Geometry check sheet. Reference: the model listing, model coordinates, mm. A direction names the side the tool comes from. Coordinates: 2 decimals unless noted, no trailing zeros. Write each loop counter-clockwise with the first axis right and the second up, starting at its lowest first coordinate (ties: lowest second). Pieces come first, ordered by that corner, then holes. Notation, with made-up numbers: (61.5, 75.5) -> (118.5, 75.5) arc R12 ccw to (118.5, 86.5) -> close; hole circle Ø3 at (63.5, -11). An arc over 180 degrees is marked (long way). Answer in a Markdown table with one row per item. Add a question column.
1. Cross-section at A-A on y = -35. Record the cut outline in (x, z).
2. Set-up check for faces 5 (the flat face through (0.737, -25, 30)), 6 (the flat face through (-1, -25, 16.398)), 7 (the flat face through (1, 0, 24)): record each of +Z, -Z, +X, -X, +Y, -Y from which the full face is reachable in a straight line by a thin tool's end or side.
3. Cross-section at D-D on x = -4. Record the cut outline in (y, z).
4. Cross-section at B-B on x = -7. Record the cut outline in (y, z).
5. Mould release check, pull along X, two halves, no side actions. Record for faces 1 (the flat face through (-6.263, -25, 5)), 2 (the cylindrical face through (-4.833, -14.549, 40.919)), 3 (the flat face through (-4, -25, 39.398)), 4 (the cylindrical face through (-6.589, -36.464, 40.919)): pulls with the +X half, pulls with the -X half, needs draft (parallel to the pull), parting line crosses it, or undercut.
6. Depth check by flat-ended pin: P1, Ø1.5, axis at y = -25, z = 36.5, coming from the -X side; P2, Ø2, axis at x = 1, y = -13, coming from the -Z side; P3, Ø2, axis at x = -4.5, z = 3, coming from the -Y side; P4, Ø18.5, axis at y = -27.5, z = 2, coming from the +X side. Enter the tip coordinate at first touch or a pass-through.
7. Cross-section at C-C on z = 5.5. Record the cut outline in (x, y).
8. Scan lines: L1, parallel to Z at x = -8.5, y = -35; L2, parallel to Z at x = -7.55, y = -15; L3, parallel to Z at x = -5, y = -9.5. Record each from-to range of solid material in increasing order. Write a range as from..to.
```python
from build123d import *

# Parameters (mm, degrees)
F1_DEPTH = 50
F2_R     = 1.5
F3_DEPTH = 10
F4_R     = 1.5
F5_DEPTH = 25


with BuildPart() as f1:
    # F0 (on Front) → F1 (new body)
    with BuildSketch(Plane.XZ):
        Polygon((-9.26335, 42.398173), (-9.26335, 39.398173), (0.73665, 39.398173), (0.73665, 19.398173), (-9.26335, 19.398173), (-9.26335, -6.901827), (-6.26335, -6.901827), (-6.26335, 16.398173), (3.73665, 16.398173), (3.73665, 42.398173), align=None)
    extrude(amount=F1_DEPTH)

    # F2 (on face) → F3 (cut)
    with BuildSketch(Plane.XY.offset(42.398173)):
        with Locations((-6.26335, -35)):
            Circle(F2_R)
        with Locations((-6.26335, -15)):
            Circle(F2_R)
    extrude(amount=-F3_DEPTH, mode=Mode.SUBTRACT)

    # F4 (on face) → F5 (cut)
    with BuildSketch(Plane.YZ.offset(-6.26335)):
        with Locations((-35, 6.098173)):
            Circle(F4_R)
        with Locations((-15, 6.098173)):
            Circle(F4_R)
    extrude(amount=-F5_DEPTH, mode=Mode.SUBTRACT)


solid = f1.part
```
Results found:
| question | item | result |
|---|---|---|
| 1 | outline | (-9.26, -6.9) -> (-6.26, -6.9) -> (-6.26, 4.6) -> (-9.26, 4.6) -> close; (-9.26, 7.6) -> (-6.26, 7.6) -> (-6.26, 16.4) -> (3.74, 16.4) -> (3.74, 42.4) -> (-4.76, 42.4) -> (-4.76, 39.4) -> (0.74, 39.4) -> (0.74, 19.4) -> (-9.26, 19.4) -> close; (-9.26, 39.4) -> (-7.76, 39.4) -> (-7.76, 42.4) -> (-9.26, 42.4) -> close |
| 2 | face 5 | -X, +Y, -Y |
| 2 | face 6 | -Z, +X, +Y, -Y |
| 2 | face 7 | +Z, -Z, +X, -X, +Y |
| 3 | outline | (-50, 16.4) -> (0, 16.4) -> (0, 19.4) -> (-50, 19.4) -> close; (-50, 39.4) -> (0, 39.4) -> (0, 42.4) -> (-50, 42.4) -> close |
| 4 | outline | (-50, -6.9) -> (0, -6.9) -> (0, 19.4) -> (-50, 19.4) -> close; (-50, 39.4) -> (-36.31, 39.4) -> (-36.31, 42.4) -> (-50, 42.4) -> close; (-33.69, 39.4) -> (-16.31, 39.4) -> (-16.31, 42.4) -> (-33.69, 42.4) -> close; (-13.69, 39.4) -> (0, 39.4) -> (0, 42.4) -> (-13.69, 42.4) -> close; hole circle Ø3 at (-35, 6.1); hole circle Ø3 at (-15, 6.1) |
| 5 | face 1 | pulls with the +X half |
| 5 | face 2 | undercut |
| 5 | face 3 | needs draft |
| 5 | face 4 | undercut |
| 6 | P1 | stops at x = 0.74 |
| 6 | P2 | stops at z = 16.4 |
| 6 | P3 | passes through |
| 6 | P4 | stops at x = -6.26 |
| 7 | outline | (-9.26, -50) -> (-6.26, -50) -> (-6.26, -36.38) -> (-9.26, -36.38) -> close; (-9.26, -33.62) -> (-6.26, -33.62) -> (-6.26, -16.38) -> (-9.26, -16.38) -> close; (-9.26, -13.62) -> (-6.26, -13.62) -> (-6.26, 0) -> (-9.26, 0) -> close |
| 8 | L1 | z = -6.9..4.6, 7.6..19.4, 39.4..42.4 |
| 8 | L2 | z = -6.9..4.6, 7.6..19.4 |
| 8 | L3 | z = 16.4..19.4, 39.4..42.4 |
